Part model, mm, in its own coordinate system. Face numbers are marked on the shaded views. A direction names the side the tool comes from. Give positions to 0.01 mm unless a question says otherwise; leave off trailing zeros. Order: outer loops, then holes, each group sorted by start corner. A loop starts at its lowest first (then second) coordinate and runs counter-clockwise, first axis right, second up. Notation, with made-up numbers: M -18,88.25 L -14,88.25 A28 ccw -14,125.25 Z; hole C -37.5,-26.75 d10. An arc over 180 degrees is marked long. Write each question's results on one line, items separated by ' | '. Start each with the question number.
from build123d import *

# Parameters (mm, degrees)
P_IDAT_VYSUNUT_M1_DEPTH  = 29
SKICA2_W                 = 21.5
SKICA2_H                 = 24.5
ODEBRAT_VYSUNUT_M1_DEPTH = 1.5
SKICA3_R                 = 1.4
ODEBRAT_VYSUNUT_M2_DEPTH = 3.5
SKICA6_W                 = 2.9
SKICA6_H                 = 4.9
SKICA6_W_2               = 7.5
SKICA6_H_2               = 2.9
ODEBRAT_VYSUNUT_M5_DEPTH = 2
ZAOBLIT1_R               = 2.5
ZAOBLIT2_R               = 2.5
SKICA10_R                = 1.9
ODEBRAT_VYSUNUT_M7_DEPTH = 17.3
SKICA20_R                = 3
ODEBRAT_VYSUNUT_M8_DEPTH = 20
ZKOSEN_1_SIZE            = 0.5
SKICA21_W                = 5
SKICA21_H                = 29
P_IDAT_VYSUNUT_M2_DEPTH  = 5
ZAOBLIT4_R               = 2.5


with BuildPart() as part:
    # Skica1 → Přidat vysunutím1 (new body)
    with BuildSketch(Plane.XY):
        Polygon((0, 0), (90.5, 0), (90.5, 17.3), (70.5, 17.3), (70.5, 5), (0, 5), align=None)
    extrude(amount=P_IDAT_VYSUNUT_M1_DEPTH)

    # Skica2 → Odebrat vysunutím1 (cut)
    with BuildSketch(Plane(origin=(0, 5, 0), x_dir=(1, 0, 0), z_dir=(0, 1, 0))):
        with Locations((13, -14.5)):
            Rectangle(SKICA2_W, SKICA2_H)
    extrude(amount=-ODEBRAT_VYSUNUT_M1_DEPTH, mode=Mode.SUBTRACT)

    # Skica3 → Odebrat vysunutím2 (cut)
    with BuildSketch(Plane(origin=(0, 3.5, 0), x_dir=(1, 0, 0), z_dir=(0, 1, 0))):
        with Locations(Location((20.8, -23.25, 0), (0, 0, 180))):
            Circle(SKICA3_R)
        with Locations(Location((5.8, -23.25, 0), (0, 0, 180))):
            Circle(SKICA3_R)
    extrude(amount=-ODEBRAT_VYSUNUT_M2_DEPTH, mode=Mode.SUBTRACT)

    # Skica6 → Odebrat vysunutím5 (cut)
    with BuildSketch(Plane(origin=(0, 3.5, 0), x_dir=(1, 0, 0), z_dir=(0, 1, 0))):
        with Locations((5.8, -6.75)):
            Rectangle(SKICA6_W, SKICA6_H)
        with Locations((20.2, -6.75)):
            Rectangle(SKICA6_W, SKICA6_H)
        with Locations((13, -24.1)):
            Rectangle(SKICA6_W_2, SKICA6_H_2)
    extrude(amount=-ODEBRAT_VYSUNUT_M5_DEPTH, mode=Mode.SUBTRACT)

    # Zaoblit1
    zaoblit1_edges = [part.edges().sort_by_distance(p)[0] for p in [
        (0, 2.5, 29),
        (0, 2.5, 0),
    ]]
    fillet(zaoblit1_edges, radius=ZAOBLIT1_R)

    # Zaoblit2
    zaoblit2_edges = [part.edges().sort_by_distance(p)[0] for p in [
        (90.5, 8.65, 29),
        (70.5, 11.15, 29),
        (70.5, 11.15, 0),
        (90.5, 8.65, 0),
    ]]
    fillet(zaoblit2_edges, radius=ZAOBLIT2_R)

    # Skica10 → Odebrat vysunutím7 (cut)
    with BuildSketch(Plane(origin=(0, 17.3, 0), x_dir=(1, 0, 0), z_dir=(0, 1, 0))):
        with Locations(Location((74.5, -4, 0), (0, 0, 180))):
            Circle(SKICA10_R)
        with Locations(Location((86.5, -4, 0), (0, 0, 180))):
            Circle(SKICA10_R)
        with Locations(Location((86.5, -25, 0), (0, 0, 270))):
            Circle(SKICA10_R)
        with Locations(Location((74.5, -25, 0), (0, 0, 270))):
            Circle(SKICA10_R)
    extrude(amount=-ODEBRAT_VYSUNUT_M7_DEPTH, mode=Mode.SUBTRACT)

    # Skica20 → Odebrat vysunutím8 (cut)
    with BuildSketch(Plane(origin=(90.5, 0, 0), x_dir=(0, 0, -1), z_dir=(1, 0, 0))):
        with Locations((-14.5, 17.3)):
            Circle(SKICA20_R)
    extrude(amount=-ODEBRAT_VYSUNUT_M8_DEPTH, mode=Mode.SUBTRACT)

    # Zkosení1
    zkosen_1_edges = [part.edges().sort_by_distance(p)[0] for p in [
        (74.5, 17.3, 23.1),
        (86.5, 17.3, 23.1),
        (88.4, 17.3, 4),
        (76.4, 17.3, 4),
    ]]
    chamfer(zkosen_1_edges, length=ZKOSEN_1_SIZE)

    # Skica21 → Přidat vysunutím2 (add)
    with BuildSketch(Plane(origin=(0, 5, 0), x_dir=(1, 0, 0), z_dir=(0, 1, 0))):
        with Locations((28.745471576, -14.5)):
            Rectangle(SKICA21_W, SKICA21_H)
    extrude(amount=P_IDAT_VYSUNUT_M2_DEPTH)

    # Zaoblit4
    zaoblit4_edges = [part.edges().sort_by_distance(p)[0] for p in [
        (28.745471576, 10, 29),
        (28.745471576, 10, 0),
    ]]
    fillet(zaoblit4_edges, radius=ZAOBLIT4_R)


solid = part.part
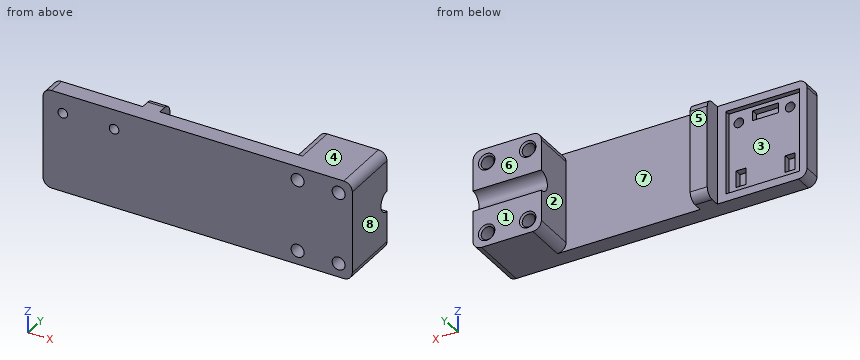
(1) Pull direction X, two halves, no side cores. Call the marked faces 6, 7 and 8: +X half, -X half, draft (parallel to the pull), parting line (faces both ways), or undercut.
(2) Drop flat-ended pins along their axis: P1, Ø8, axis at x = 42, z = 19.5, coming from the +Y side; P2, Ø8, axis at y = 10.5, z = 4, coming from the -X side. Give the stop position or say it passes through.
(3) Tool access for the marked faces 1, 2, 3, 4 and 5: list every direction of +Z, -Z, +X, -X, +Y, -Y with a clear straight run to the whole face (end or side of a thin tool).
(4) Saw through at D-D on x = 86.5. Give the cut face in (y, z).
(5) Saw through at C-C on z = 20.75. Give the cut face in (x, y).
(6) Probe L1, parallel to X at y = 10.5, z = 25; L2, parallel to Z at x = 74.5, y = 10; L3, parallel to Z at x = 20.8, y = 2.8. List the from-to ranges inside material, lowest first.
(7) Saw through at B-B on x = 20.8. Give the cut face in (y, z), plus the area to 4 significant figures.
(8) Saw through at A-A on y = 6.25. Give the cut face in (x, z).
Taken from the geometry:
1) face 6: draft | face 7: undercut | face 8: +X half
2) P1: stops at y = 5 | P2: stops at x = 26.25
3) face 1: +Z, -Z, +X, -X, +Y | face 2: +Z, -Z, +Y | face 3: +Y | face 4: +Z, +X, -X, +Y, -Y | face 5: +Z, -Z, -X, +Y
4) outline: M 0,0 L 17.3,0 L 17.3,1.6 L 16.8,2.1 L 0,2.1 Z; M 0,5.9 L 16.8,5.9 L 17.3,6.4 L 17.3,11.5 A3 cw 17.3,17.5 L 17.3,22.6 L 16.8,23.1 L 0,23.1 Z; M 0,26.9 L 16.8,26.9 L 17.3,27.4 L 17.3,29 L 0,29 Z
5) outline: M 0,0 L 90.5,0 L 90.5,17.3 L 70.5,17.3 L 70.5,5 L 31.25,5 L 31.25,10 L 26.25,10 L 26.25,5 L 23.75,5 L 23.75,3.5 L 2.25,3.5 L 2.25,5 L 0,5 Z
6) L1: x = 70.5 to 72.6, 76.4 to 84.6, 88.4 to 90.5 | L2: z = 0 to 2.1, 5.9 to 23.1, 26.9 to 29 | L3: z = 0 to 4.3, 9.2 to 21.85, 24.65 to 29
7) outline: M 0,0 L 5,0 L 5,2.25 L 3.5,2.25 L 3.5,4.3 L 1.5,4.3 L 1.5,9.2 L 3.5,9.2 L 3.5,21.85 L 0,21.85 Z; M 0,24.65 L 3.5,24.65 L 3.5,26.75 L 5,26.75 L 5,29 L 0,29 Z | area: 88.65 mm²
8) outline: M 26.25,0 L 31.25,0 L 31.25,29 L 26.25,29 Z; M 70.5,2.5 A2.5 ccw 73,0 L 88,0 A2.5 ccw 90.5,2.5 L 90.5,26.5 A2.5 ccw 88,29 L 73,29 A2.5 ccw 70.5,26.5 Z; hole C 74.5,4 d3.8; hole C 74.5,25 d3.8; hole C 86.5,4 d3.8; hole C 86.5,25 d3.8
